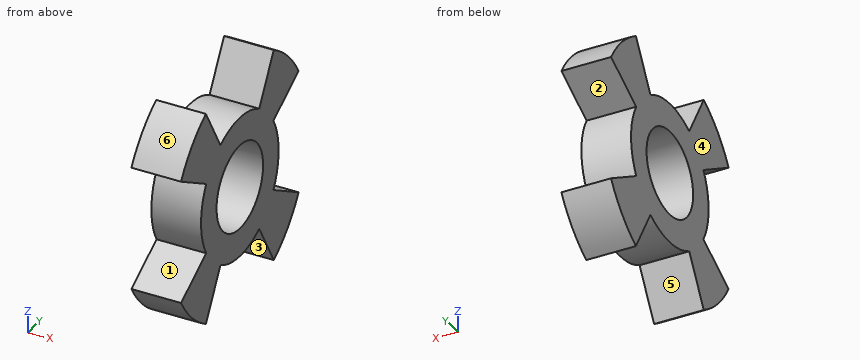
```python
from build123d import *

# Parameters (mm, degrees)
SKETCH1_R               = 35
BOSS_EXTRUDE1_DEPTH     = 14
CUT_EXTRUDE1_DEPTH      = 52.439284598
CUT_EXTRUDE2_DEPTH      = 46.094345544
CUT_EXTRUDE2_DEPTH_BACK = 46.094345544
SKETCH3_R               = 12


with BuildPart() as part:
    # Sketch1 → Boss-Extrude1 (new body)
    with BuildSketch(Plane(origin=(0, 0, 0), x_dir=(0, 0, -1), z_dir=(1, 0, 0))):
        Circle(SKETCH1_R)
    extrude(amount=BOSS_EXTRUDE1_DEPTH)

    # Sketch2 → Cut-Extrude1 (cut, through all)
    with BuildSketch(Plane(origin=(0, 0, 0), x_dir=(0, 0, -1), z_dir=(1, 0, 0))):
        with BuildLine():
            Line((-17.5, 30.310889132), (-10, 17.320508076))
            ThreePointArc((-10, 17.320508076), (0, 20), (10, 17.320508076))
            Line((10, 17.320508076), (17.5, 30.310889132))
            ThreePointArc((17.5, 30.310889132), (0, 35), (-17.5, 30.310889132))
        make_face()
        with BuildLine():
            Line((30.310889132, 17.5), (17.320508076, 10))
            ThreePointArc((17.320508076, 10), (20, 0), (17.320508076, -10))
            Line((17.320508076, -10), (30.310889132, -17.5))
            ThreePointArc((30.310889132, -17.5), (35, 0), (30.310889132, 17.5))
        make_face()
        with BuildLine():
            Line((17.5, -30.310889132), (10, -17.320508076))
            ThreePointArc((10, -17.320508076), (0, -20), (-10, -17.320508076))
            Line((-10, -17.320508076), (-17.5, -30.310889132))
            ThreePointArc((-17.5, -30.310889132), (0, -35), (17.5, -30.310889132))
        make_face()
        with BuildLine():
            Line((-30.310889132, -17.5), (-17.320508076, -10))
            ThreePointArc((-17.320508076, -10), (-20, 0), (-17.320508076, 10))
            Line((-17.320508076, 10), (-30.310889132, 17.5))
            ThreePointArc((-30.310889132, 17.5), (-35, 0), (-30.310889132, -17.5))
        make_face()
    extrude(amount=CUT_EXTRUDE1_DEPTH, mode=Mode.SUBTRACT)

    # Sketch3 → Cut-Extrude2 (cut, two sides: drawn at the far end of the back side and taken through both)
    with BuildSketch(Plane(origin=(0, 0, 0), x_dir=(0, 0, -1), z_dir=(1, 0, 0)).offset(-CUT_EXTRUDE2_DEPTH_BACK)):
        Circle(SKETCH3_R)
    extrude(amount=CUT_EXTRUDE2_DEPTH + CUT_EXTRUDE2_DEPTH_BACK, mode=Mode.SUBTRACT)


solid = part.part
```
Geometry check sheet. Reference: the model listing, model coordinates, mm. Face numbers are marked on the shaded views. A direction names the side the tool comes from. Coordinates: 2 decimals unless noted, no trailing zeros. Order: outer loops, then holes, each group sorted by start corner. A loop starts at its lowest first (then second) coordinate and runs counter-clockwise, first axis right, second up. Notation, with made-up numbers: M 0,49.5 L 34,49.5 A21 cw 34,83.5 Z; hole C -19,17.25 d6. An arc over 180 degrees is marked long. Answer as a JSON object with one key per item and string values.
Q1. Scan lines: line 1 (Z direction, x = 12, y = 0); line 2 (Y direction, x = 8.25, z = 18). Record each from-to range of solid material in increasing order.
Results are:
{"line 1": "z = -20 to -12, 12 to 20", "line 2": "y = -30.02 to -10.39, -8.72 to 8.72, 10.39 to 30.02"}
Q2. Cross-section at D-D on y = -19. Record the cut outline in (x, z) (3 decimals).
Results are:
{"outline": "M 0,-29.394 L 14,-29.394 L 14,-10.97 L 0,-10.97 Z; M 0,-6.245 L 14,-6.245 L 14,6.245 L 0,6.245 Z; M 0,10.97 L 14,10.97 L 14,29.394 L 0,29.394 Z"}
Q3. Tool access check on the marked faces 1, 2 and 3. Record the directions out of +Z, -Z, +X, -X, +Y, -Y that give a thin tool (end or side, any length) a straight path to the whole face; none if there is none.
Results are:
{"face 1": "+X, -X, -Y", "face 2": "+X, -X, +Y", "face 3": "-Z, +X, -X"}
Q4. Cross-section at A-A on y = 0. Record the cut outline in (x, z), and give its area (3 significant figures).
Results are:
{"outline": "M 0,-20 L 14,-20 L 14,-12 L 0,-12 Z; M 0,12 L 14,12 L 14,20 L 0,20 Z", "area": "224 mm²"}
Q5. Cross-section at C-C on x = 3.5. Record the cut outline in (y, z).
Results are:
{"outline": "M -30.31,-17.5 A35 ccw -17.5,-30.31 L -10,-17.32 A20 ccw 10,-17.32 L 17.5,-30.31 A35 ccw 30.31,-17.5 L 17.32,-10 A20 ccw 17.32,10 L 30.31,17.5 A35 ccw 17.5,30.31 L 10,17.32 A20 ccw -10,17.32 L -17.5,30.31 A35 ccw -30.31,17.5 L -17.32,10 A20 ccw -17.32,-10 Z; hole C 0,0 d24"}
Q6. Depth check by flat-ended pin: pin 1 Ø2 at (x, z) = (5.5, 2) entering from -Y (3 decimals); pin 2 Ø21.5 at (y, z) = (0, 0) entering from -X; pin 3 Ø4 at (x, z) = (6, -20) entering from +Y. Enter the tip coordinate at first touch or a pass-through.
Results are:
{"pin 1": "stops at y = -19.975", "pin 2": "passes through", "pin 3": "stops at y = 30.02"}
Q7. Release check for a two-part mould opening along Y. For the marked faces 4, 5 and 6 record: released by +Y, released by -Y, zero draft, split by the parting line, or undercut.
Results are:
{"face 4": "zero draft", "face 5": "undercut", "face 6": "released by -Y"}
